Work out the finished part from the listing and answer in its coordinate system (mm). A direction names the side the tool comes from. Coordinates: 2 decimals unless noted, no trailing zeros. Order: outer loops, then holes, each group sorted by start corner. A loop starts at its lowest first (then second) coordinate and runs counter-clockwise, first axis right, second up.
1. The part is cut by section B-B, the plane z = 29.5. Give the vertices of the cut face in (x, y).
2. The part is cut by section A-A, the plane y = -2.25. Give the vertices of the cut face in (x, z).
3. A tool of negligible diameter and unlimited length cuts with its end or side. For faces 4 (the flat face through (-101.6, -3, 44)), 5 (the flat face through (69, 0, 45)), 6 (the flat face through (0, -3, 12.7)), from which of +Z, -Z, +X, -X, +Y, -Y can it reach the whole face along a straight path? Write none if from no direction.
4. Flat-ended cylindrical pins translate along their axes: pin 1 Ø3.5 at (x, y) = (181.5, -10) entering from -Z; pin 2 Ø5 at (y, z) = (-2.5, 35) entering from +X; pin 3 Ø3 at (y, z) = (-6, 61) entering from -X; pin 4 Ø1.9 at (y, z) = (-1.5, 37.5) entering from -X. Find the tip coordinate at first contact, or state that the pin passes through.
5. Find the intervals of material crossed by probe 1 along Z at (x, y) = (-99, -3); probe 2 along X at (y, z) = (-5.5, 70); probe 3 along X at (y, z) = (-5.75, 19.5), in increasing order.
6. The part is cut by section C-C, the plane x = -115.5. Give the vertices of the cut face in (y, z), then the cut area to 3 significant figures.
7. Determine the mould class of faces 1 (the flat face through (-142, -3, 12.7)), 2 (the flat face through (-177.89, -6.44, 38.63)), 3 (the flat face through (-38.1, -3, 44)) for opening direction X: +X half, -X half, draft (parallel to the pull), parting line (faces both ways), or undercut.
```python
from build123d import *

# Parameters (mm, degrees)
F0_W      = 368.3
F0_H      = 76.2
F1_DEPTH  = 12.7
F2_W      = 6.35
F2_H      = 6.35
F3_DEPTH  = 368.301
F5_DEPTH  = 76.201
F6_W      = 6.35
F6_H      = 63.5
F7_DEPTH  = 6.35
F8_W      = 7.000554
F8_H      = 6.35
F9_DEPTH  = 260.428428
F10_W     = 6.35
F10_H     = 6.35
F11_DEPTH = 260.428428


with BuildPart() as f1:
    # F0 (on Front) → F1 (new body)
    with BuildSketch(Plane.XZ):
        with Locations((0, 38.1)):
            Rectangle(F0_W, F0_H)
    extrude(amount=F1_DEPTH)

    # F2 (on face) → F3 (cut, through all)
    with BuildSketch(Plane.YZ.offset(184.15)):
        with Locations((-3.175, 9.525)):
            Rectangle(F2_W, F2_H)
    extrude(amount=-F3_DEPTH, mode=Mode.SUBTRACT)

    # F4 (on face) → F5 (cut, through all)
    with BuildSketch(Plane.XY.offset(76.2)):
        Polygon((-184.15, 0), (-184.15, -12.7), (-171.45, 0), align=None)
        Polygon((184.15, -12.7), (184.15, 0), (171.45, 0), align=None)
    extrude(amount=-F5_DEPTH, mode=Mode.SUBTRACT)

    # F6 (on face) → F7 (cut)
    with BuildSketch(Plane(origin=(0, 0, 0), x_dir=(-1, 0, 0), z_dir=(0, 1, 0))):
        with Locations((-104.775, 44.45)):
            Rectangle(F6_W, F6_H)
        with Locations((-34.925, 44.45)):
            Rectangle(F6_W, F6_H)
        with Locations((34.925, 44.45)):
            Rectangle(F6_W, F6_H)
        with Locations((104.775, 44.45)):
            Rectangle(F6_W, F6_H)
    extrude(amount=-F7_DEPTH, mode=Mode.SUBTRACT)

    # F8 (on face) → F9 (cut, through all)
    with BuildSketch(Plane(origin=(-85.725, 85.725, 0), x_dir=(-0.707107, -0.707107, 0), z_dir=(-0.707107, 0.707107, 0))):
        with Locations((135.693693, 53.975)):
            Rectangle(F8_W, F8_H)
        with Locations((135.693693, 22.225)):
            Rectangle(F8_W, F8_H)
    extrude(amount=-F9_DEPTH, mode=Mode.SUBTRACT)

    # F10 (on face) → F11 (cut, through all)
    with BuildSketch(Plane(origin=(85.725, 85.725, 0), x_dir=(-0.707107, 0.707107, 0), z_dir=(0.707107, 0.707107, 0))):
        with Locations((-136.01897, 53.975)):
            Rectangle(F10_W, F10_H)
        with Locations((-136.01897, 22.225)):
            Rectangle(F10_W, F10_H)
    extrude(amount=-F11_DEPTH, mode=Mode.SUBTRACT)


solid = f1.part
```
Geometry says:
1. outline: (-184.15, -12.7) - (184.15, -12.7) - (171.45, 0) - (107.95, 0) - (107.95, -6.35) - (101.6, -6.35) - (101.6, 0) - (38.1, 0) - (38.1, -6.35) - (31.75, -6.35) - (31.75, 0) - (-31.75, 0) - (-31.75, -6.35) - (-38.1, -6.35) - (-38.1, 0) - (-101.6, 0) - (-101.6, -6.35) - (-107.95, -6.35) - (-107.95, 0) - (-171.45, 0) - close
2. outline: (-173.7, 0) - (173.7, 0) - (173.7, 6.35) - (-173.7, 6.35) - close; (-173.7, 12.7) - (-107.95, 12.7) - (-107.95, 76.2) - (-173.7, 76.2) - close; (-101.6, 12.7) - (-38.1, 12.7) - (-38.1, 76.2) - (-101.6, 76.2) - close; (-31.75, 12.7) - (31.75, 12.7) - (31.75, 76.2) - (-31.75, 76.2) - close; (38.1, 12.7) - (101.6, 12.7) - (101.6, 76.2) - (38.1, 76.2) - close; (107.95, 12.7) - (173.7, 12.7) - (173.7, 76.2) - (107.95, 76.2) - close
3. face 4: +Z, +Y
3. face 5: +Z, -Z, +X, -X, +Y
3. face 6: +X, -X, +Y
4. pin 1: stops at z = 0
4. pin 2: stops at x = 176.45
4. pin 3: stops at x = -178.95
4. pin 4: stops at x = -173.9
5. probe 1: z = 0 to 6.35, 12.7 to 76.2
5. probe 2: x = -176.95 to -107.95, -101.6 to -38.1, -31.75 to 31.75, 38.1 to 101.6, 107.95 to 176.95
5. probe 3: x = -177.2 to -107.95, -101.6 to -38.1, -31.75 to 31.75, 38.1 to 101.6, 107.95 to 177.2
6. outline: (-12.7, 0) - (0, 0) - (0, 6.35) - (-6.35, 6.35) - (-6.35, 12.7) - (0, 12.7) - (0, 76.2) - (-12.7, 76.2) - close
6. area: 927 mm2
7. face 1: draft
7. face 2: -X half
7. face 3: undercut
